from build123d import *

# Parameters (mm, degrees)
F0_W     = 42
F0_H     = 39
F1_DEPTH = 3
F0_H_2   = 3
F2_DEPTH = 45
F4_D     = 5
F6_D     = 5
F7_R     = 12
F8_DEPTH = 25


with BuildPart() as f1:
    # F0 (on Top) → F1 (new body)
    with BuildSketch(Plane.XY):
        with Locations((0, 1.5)):
            Rectangle(F0_W, F0_H)
    extrude(amount=F1_DEPTH)

    # F0 (on Top) → F2 (join)
    with BuildSketch(Plane.XY):
        with Locations((0, -19.5)):
            Rectangle(F0_W, F0_H_2)
    extrude(amount=F2_DEPTH)

    # F4 (through all)
    with Locations(Plane.XY.offset(3)):
        with Locations((10, -9), (10, 11), (-10, 11), (-10, -9)):
            Hole(F4_D / 2)

    # F6 (through all)
    with Locations(Plane(origin=(0, -18, 0), x_dir=(-1, 0, 0), z_dir=(0, 1, 0))):
        with Locations((-15.5, 39.5), (-15.5, 8.5), (15.5, 8.5), (15.5, 39.5)):
            Hole(F6_D / 2)

    # F7 (on face) → F8 (cut)
    with BuildSketch(Plane(origin=(0, -18, 0), x_dir=(-1, 0, 0), z_dir=(0, 1, 0))):
        with Locations((0, 24)):
            Circle(F7_R)
    extrude(amount=-F8_DEPTH, mode=Mode.SUBTRACT)


solid = f1.part
Could you check a few things on this model? Use its own coordinates, in mm. A direction names the side the tool comes from. Coordinates: 2 decimals unless noted, no trailing zeros. Write each loop counter-clockwise with the first axis right and the second up, starting at its lowest first coordinate (ties: lowest second). Pieces come first, ordered by that corner, then holes. Notation, with made-up numbers: (10, 39) - (38, 39) arc R14 cw to (38, 47) - close; hole circle Ø2 at (-15.5, 40). An arc over 180 degrees is marked (long way). Put each result on its own line as item: value. Start each with the question number.
Q1. I want a section at D-D on x = 15.5. Write out the boundary of the cut face in (y, z), plus the area to 3 significant figures.
Q2. I want a section at A-A on y = 11. Write out the boundary of the cut face in (x, z), plus the area to 3 significant figures.
Q3. Please list where these lines run through material, in increasing order: L1, parallel to Y at x = 10, z = 1.65; L2, parallel to Z at x = 15.5, y = -19.3; L3, parallel to X at y = -19, z = 39.
Q4. Thinking about a two-plate mould opening in Z: for faces 3 (the cylindrical face through (14.96, -19.52, 37.06)), 4 (the flat face through (0, 0, 0)), 5 (the flat face through (21, -19, 12)), 6 (the flat face through (0, 2, 3)), which applies, pulls with the +Z half, pulls with the -Z half, needs draft (parallel to the pull), parting line crosses it, or undercut?
Q5. I want a section at C-C on x = 1. Write out the boundary of the cut face in (y, z).
Q6. Which directions (+Z, -Z, +X, -X, +Y, -Y) give clear straight access to the entire face, cutting with the end or side of a thin tool? Please do faces 1 (the cylindrical face through (-9.46, 8.56, 1.48)), 2 (the flat face through (9, -18, 33)).
Q7. I want a section at B-B on z = 39.5. Write out the boundary of the cut face in (x, y), plus the area to 3 significant figures.
Q8. I'm going to push a flat-ended pin straight in: P1, Ø6, axis at x = -10, y = -9, coming from the +Z side. Where does the tip first touch, or does it pass through?
Checks:
1. outline: (-21, 0) - (21, 0) - (21, 3) - (-18, 3) - (-18, 6) - (-21, 6) - close; (-21, 11) - (-18, 11) - (-18, 37) - (-21, 37) - close; (-21, 42) - (-18, 42) - (-18, 45) - (-21, 45) - close
1. area: 222 mm²
2. outline: (-21, 0) - (-12.5, 0) - (-12.5, 3) - (-21, 3) - close; (-7.5, 0) - (7.5, 0) - (7.5, 3) - (-7.5, 3) - close; (12.5, 0) - (21, 0) - (21, 3) - (12.5, 3) - close
2. area: 96.0 mm²
3. L1: -21 to -11.5, -6.5 to 8.5, 13.5 to 21
3. L2: 0 to 6, 11 to 37, 42 to 45
3. L3: -21 to -17.95, -13.05 to 13.05, 17.95 to 21
4. face 3: undercut
4. face 4: pulls with the -Z half
4. face 5: needs draft
4. face 6: pulls with the +Z half
5. outline: (-21, 0) - (21, 0) - (21, 3) - (-18, 3) - (-18, 12.04) - (-21, 12.04) - close; (-21, 35.96) - (-18, 35.96) - (-18, 45) - (-21, 45) - close
6. face 1: +Z, -Z
6. face 2: +Z, +X, -X, +Y
7. outline: (-21, -21) - (-18, -21) - (-18, -18) - (-21, -18) - close; (-13, -21) - (13, -21) - (13, -18) - (-13, -18) - close; (18, -21) - (21, -21) - (21, -18) - (18, -18) - close
7. area: 96.0 mm²
8. P1: z = 3
